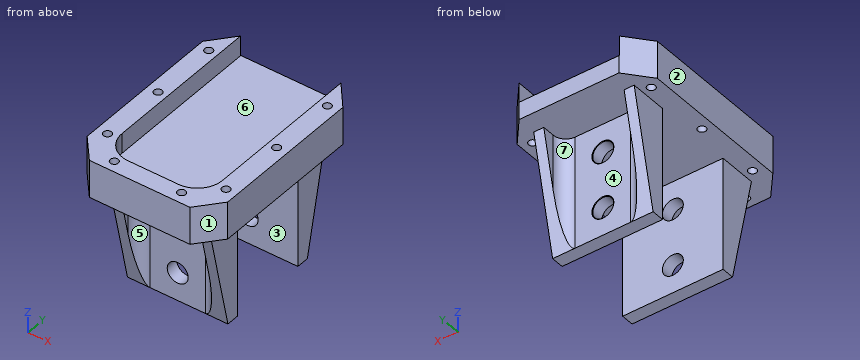
from build123d import *

# Parameters (mm, degrees)
SKETCH1_W                      = 35.56
SKETCH1_H                      = 50.8
BOSS_EXTRUDE1_DEPTH            = 9.525
SKETCH2_W                      = 25.4
SKETCH2_H                      = 46.22
CUT_EXTRUDE2_DEPTH             = 5.08
TAP_DRILL_FOR_M2_5X0_45_TAP1_D = 2.05
SKETCH13_W                     = 25.4
SKETCH13_H                     = 3.175
BOSS_EXTRUDE2_DEPTH            = 28.575
CUT_EXTRUDE3_DEPTH             = 73.778867812
FILLET1_R                      = 6.35
M5_CLEARANCE_HOLE1_D           = 5.3
M5_CLEARANCE_HOLE1_CSINK_D     = 5.55
M5_CLEARANCE_HOLE1_CSINK_ANGLE = 90
RIB7_REACH                     = 67.774
SKETCH14_WALL_W                = 162.819779212
SKETCH14_WALL_H                = 2.54
RIB8_START                     = -2.54
RIB8_DEPTH                     = 2.54
RIB9_REACH                     = 67.774
SKETCH17_WALL_W                = 162.819779212
SKETCH17_WALL_H                = 2.54
RIB10_START                    = -2.54
RIB10_DEPTH                    = 2.54
FILLET2_R                      = 3.175
FILLET3_R                      = 3.175


# Read off the part's stored shape, not the designer's step: Rib8, Rib10
with BuildPart() as part:
    # Sketch1 → Boss-Extrude1 (new body)
    with BuildSketch(Plane.XY):
        with Locations((-17.78, 25.4)):
            Rectangle(SKETCH1_W, SKETCH1_H)
    extrude(amount=BOSS_EXTRUDE1_DEPTH)

    # Sketch2 → Cut-Extrude2 (cut)
    with BuildSketch(Plane.XY.offset(9.525)):
        with Locations((-17.78, 27.69)):
            Rectangle(SKETCH2_W, SKETCH2_H)
    extrude(amount=-CUT_EXTRUDE2_DEPTH, mode=Mode.SUBTRACT)

    # Tap Drill for M2.5x0.45 Tap1 (through all)
    with Locations(Plane(origin=(0, 0, 0), x_dir=(-1, 0, 0), z_dir=(0, 0, -1))):
        with Locations((2.792369004, 43.087106138), (2.792369004, 26.092979092), (2.792369004, 9.105182099), (9.290740849, 2.822744672), (26.292369004, 2.787106138), (32.780032006, 9.105182099), (32.792369004, 26.087106138), (32.792369004, 43.087106138)):
            Hole(TAP_DRILL_FOR_M2_5X0_45_TAP1_D / 2)

    # Sketch13 → Boss-Extrude2 (add)
    with BuildSketch(Plane(origin=(0, 0, 0), x_dir=(-1, 0, 0), z_dir=(0, 0, -1))):
        with Locations((17.78, 37.827545037)):
            Rectangle(SKETCH13_W, SKETCH13_H)
        with Locations((17.78, 14.352545037)):
            Rectangle(SKETCH13_W, SKETCH13_H)
    extrude(amount=BOSS_EXTRUDE2_DEPTH)

    # Sketch8 → Cut-Extrude3 (cut, through all)
    with BuildSketch(Plane.XY.offset(9.525)):
        Polygon((-5.178964387, 50.8), (0, 44.591495864), (0, 50.8), align=None)
        Polygon((-35.56, 44.706622517), (-35.56, 50.8), (-30.402645731, 50.8), align=None)
        Polygon((-35.56, 5.970049098), (-35.56, 0), (-30.492594088, 0), align=None)
        Polygon((-5.092594088, -0.031324356), (0, 0), (0, 5.970049098), align=None)
    extrude(amount=-CUT_EXTRUDE3_DEPTH, mode=Mode.SUBTRACT)

    # Fillet1
    fillet1_edges = [part.edges().sort_by_distance(p)[0] for p in [
        (-30.48, 4.58, 6.985),
        (-5.08, 4.58, 6.985),
    ]]
    fillet(fillet1_edges, radius=FILLET1_R)

    # M5 Clearance Hole1 (through all)
    with Locations(Plane(origin=(-17.78, 39.415045037, -7.14375), x_dir=(0, 0, 1), z_dir=(0, 1, 0))):
        with Locations((0, 0), (-14.2875, 0)):
            CounterSinkHole(M5_CLEARANCE_HOLE1_D / 2, M5_CLEARANCE_HOLE1_CSINK_D / 2, counter_sink_angle=M5_CLEARANCE_HOLE1_CSINK_ANGLE)

    # Sketch14 wall → Rib7 (add, up to next)
    with BuildSketch(Plane(origin=(-30.48, 9.590045037, -14.2875), x_dir=(0, -0.216930457819, 0.976187060184), z_dir=(0, 0.976187060184, 0.216930457819)), mode=Mode.PRIVATE) as rib7_sk1:
        with Locations((0, 1.27)):
            Rectangle(SKETCH14_WALL_W, SKETCH14_WALL_H)
    rib7_tool1 = extrude(rib7_sk1.sketch, amount=RIB7_REACH, mode=Mode.PRIVATE) - part.part
    add(rib7_tool1.solids().sort_by_distance((-30.48, 9.590045037, -14.2875))[0])

    # Rib8 outline → Rib8 (add)
    with BuildSketch(Plane(origin=(-5.08, 0, 0), x_dir=(0, 0, -1), z_dir=(1, 0, 0)).offset(RIB8_START)):
        Polygon((0, 6.415045037), (28.575, 12.765045037), (0, 12.765045037), align=None)
    extrude(amount=RIB8_DEPTH)

    # Sketch17 wall → Rib9 (add, up to next)
    with BuildSketch(Plane(origin=(-5.08, 42.590045037, -14.2875), x_dir=(0, 0.216930457819, 0.976187060184), z_dir=(0, -0.976187060184, 0.216930457819)), mode=Mode.PRIVATE) as rib9_sk1:
        with Locations((0, 1.27)):
            Rectangle(SKETCH17_WALL_W, SKETCH17_WALL_H)
    rib9_tool1 = extrude(rib9_sk1.sketch, amount=RIB9_REACH, mode=Mode.PRIVATE) - part.part
    add(rib9_tool1.solids().sort_by_distance((-5.08, 42.590045037, -14.2875))[0])

    # Rib10 outline → Rib10 (add)
    with BuildSketch(Plane.ZY.offset(30.48).offset(RIB10_START)):
        Polygon((0, 45.765045037), (-28.575, 39.415045037), (0, 39.415045037), align=None)
    extrude(amount=RIB10_DEPTH)

    # Fillet2
    fillet2_edges = [part.edges().sort_by_distance(p)[0] for p in [
        (-27.94, 12.765045037, -14.2875),
        (-7.62, 12.765045037, -14.2875),
    ]]
    fillet(fillet2_edges, radius=FILLET2_R)

    # Fillet3
    fillet3_edges = [part.edges().sort_by_distance(p)[0] for p in [
        (-7.62, 39.415045037, -14.2875),
        (-27.94, 39.415045037, -14.2875),
    ]]
    fillet(fillet3_edges, radius=FILLET3_R)


solid = part.part
Geometry check sheet. Reference: the model listing, model coordinates, mm. Face numbers are marked on the shaded views. A direction names the side the tool comes from. Give positions to 0.01 mm unless a question says otherwise; leave off trailing zeros. Order: outer loops, then holes, each group sorted by start corner. A loop starts at its lowest first (then second) coordinate and runs counter-clockwise, first axis right, second up.
1) Draft check along Y on the marked faces 1, 2, 3 and 4. Enter one of: released by +Y, released by -Y, zero draft, split by the parting line, or undercut.
Results are:
face 1: released by -Y
face 2: zero draft
face 3: undercut
face 4: released by +Y
2) Material ranges on probe 1 along Z at (x, y) = (-17.78, 37.1) (3 decimals); probe 2 along Y at (x, z) = (-11, -26); probe 3 along X at (y, z) = (9, 7), recorded low to high.
Results are:
probe 1: z = -28.575 to -24.081, -18.781 to -9.794, -4.494 to 4.445
probe 2: y = 12.77 to 15.94, 36.24 to 39.42
probe 3: x = -35.56 to -33.8, -31.76 to -30.18, -5.38 to -3.81, -1.77 to 0
3) Cross-section at A-A (x = -17.78). Give the number of separate pieces and of enclosed holes in the cut face, then the cut area to 3 significant figures.
Results are:
separate pieces: 5
enclosed holes: 0
area: 363 mm2
4) Cross-section at B-B (z = -25). Record the boundary of the cut face in (x, y) (3 decimals).
Results are:
outline: (-30.48, 11.971) - (-26.866, 11.971) arc R3.175 cw to (-24.765, 12.765) - (-10.795, 12.765) arc R3.175 cw to (-8.694, 11.971) - (-5.08, 11.971) - (-5.08, 15.94) - (-30.48, 15.94) - close; (-30.48, 36.24) - (-5.08, 36.24) - (-5.08, 40.209) - (-8.694, 40.209) arc R3.175 cw to (-10.795, 39.415) - (-24.765, 39.415) arc R3.175 cw to (-26.866, 40.209) - (-30.48, 40.209) - close
5) Gauge pin test, flat ends, axial feed: pin 1 (2.5 mm diameter, centred on x = -32.79, y = 26.09, fed in from +Z) (3 decimals); pin 2 (8.5 mm diameter, centred on x = -17.78, z = -7.14, fed in from +Y); pin 3 (3 mm diameter, centred on y = 11.5, z = -13, fed in from -X); pin 4 (1.5 mm diameter, centred on x = -10, y = 31.5, fed in from -Z). Record the tip position at first contact, or that the pin passes through.
Results are:
pin 1: stops at z = 9.525
pin 2: stops at y = 39.42
pin 3: stops at x = -30.48
pin 4: stops at z = 0
6) Tool access check on the marked faces 5, 6 and 7. Record the directions out of +Z, -Z, +X, -X, +Y, -Y that give a thin tool (end or side, any length) a straight path to the whole face; none if there is none.
Results are:
face 5: -Z, -Y
face 6: +Z, +Y
face 7: -Z, +Y
7) Cross-section at C-C (y = 19.5). Record the boundary of the cut face in (x, z) (3 decimals), then the cut area to 3 significant figures.
Results are:
outline: (-35.56, 0) - (0, 0) - (0, 9.525) - (-5.08, 9.525) - (-5.08, 4.445) - (-30.48, 4.445) - (-30.48, 9.525) - (-35.56, 9.525) - close
area: 210 mm2
